Solid Edge part; units mm, degrees
sketch "Sketch1" plane through (0, 0, 0) normal (0, 0, 1) x (1, 0, 0)
  line L0 (0, 0) -> (115, 0)
  line L1 (115, 0) -> (115, 215)
  line L2 (115, 215) -> (0, 215)
  line L3 (0, 215) -> (0, 0)
  dimension "D1" = 115
  dimension "D2" = 0
extrude "Protrusion1" add sketch "Sketch1" along normal blind 30
sketch "Sketch2" plane through (57.5, 107.5, 30) normal (0, 0, 1) x (1, 0, 0)
  circle A0 centre (-20.8, 60.05) radius 30
extrude "ExtrudedCutout_1" cut sketch "Sketch2" against normal blind 2
sketch "Sketch3" plane through (57.5, 107.5, 0) normal (0, 0, -1) x (0, 1, 0)
  circle A0 centre (-75, -25) radius 2
  circle A1 centre (75, -25) radius 2
  circle A2 centre (75, 25) radius 2
  circle A3 centre (-75, 25) radius 2
  dimension "D1" = 75
  dimension "D2" = 75
extrude "ExtrudedCutout_2" cut sketch "Sketch3" against normal blind 3
sketch "Sketch4" plane through (57.5, 107.5, 30) normal (0, 0, 1) x (0, 1, 0)
  line L0 (-107.5, -54.5317) -> (-93.8266, -54.5317)
  line L1 (-93.8266, -54.5317) -> (-93.8266, 35.8867)
  line L2 (-93.8266, 35.8867) -> (-107.5, 35.8867)
  line L3 (-107.5, 35.8867) -> (-107.5, -54.5317)
extrude "ExtrudedCutout_3" cut sketch "Sketch4" against normal blind 11.4081
sketch "Sketch5" plane through (115, 107.5, 15) normal (1, 0, 0) x (0, 1, 0)
  circle A0 centre (-75, -2.5) radius 2
  circle A1 centre (75, -2.5) radius 2
extrude "ExtrudedCutout_4" cut sketch "Sketch5" against normal blind 5
mirror "Mirror1" about plane through (57.5, 0, 0) normal (1, 0, 0) of "ExtrudedCutout_4"
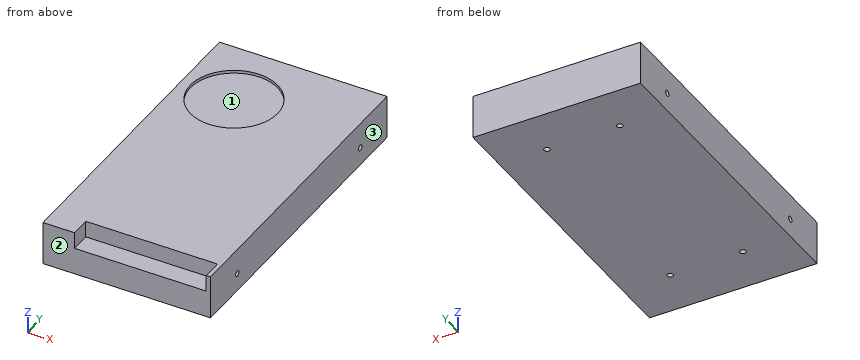
Part model, mm, in its own coordinate system. Face numbers are marked on the shaded views. Round coordinates to 2 decimals unless told otherwise and drop trailing zeros. Write each loop counter-clockwise with the first axis right and the second up, starting at its lowest first coordinate (ties: lowest second). Pieces come first, ordered by that corner, then holes.
Item 1: Cut at A-A, the plane x = 36.7. Give the cut face in (y, z), plus the area to 3 significant figures.
Results:
outline: (0, 0) - (215, 0) - (215, 30) - (197.55, 30) - (197.55, 28) - (137.55, 28) - (137.55, 30) - (13.67, 30) - (13.67, 18.59) - (0, 18.59) - close
area: 6,170 mm2
Item 2: Drop flat-ended pins along their axis: pin 1 Ø1.2 at (y, z) = (31.5, 12.5) entering from +X; pin 2 Ø3 at (x, y) = (32.5, 32.5) entering from -Z; pin 3 Ø11 at (x, y) = (50.5, 4) entering from +Z. Give the stop position or say it passes through.
Results:
pin 1: stops at x = 110
pin 2: stops at z = 3
pin 3: stops at z = 18.59
Item 3: Cut at C-C, the plane x = 76.5. Give the cut face in (y, z), plus the area to 3 significant figures.
Results:
outline: (0, 0) - (215, 0) - (215, 30) - (13.67, 30) - (13.67, 18.59) - (0, 18.59) - close
area: 6,290 mm2
Item 4: Two-plate mould, pull along X, no slides. Class the marked faces 1, 2 and 3: +X half, -X half, draft (parallel to the pull), parting line (faces both ways), or undercut.
Results:
face 1: undercut
face 2: draft
face 3: +X half
Item 5: Cut at B-B, the plane y = 167.55. Give the cut face in (x, z).
Results:
outline: (0, 0) - (115, 0) - (115, 30) - (66.7, 30) - (66.7, 28) - (6.7, 28) - (6.7, 30) - (0, 30) - close
Item 6: Cut at D-D, the plane y = 32.5. Give the cut face in (x, z), plus the area to 3 significant figures.
Results:
outline: (0, 0) - (30.5, 0) - (30.5, 3) - (34.5, 3) - (34.5, 0) - (80.5, 0) - (80.5, 3) - (84.5, 3) - (84.5, 0) - (115, 0) - (115, 10.5) - (110, 10.5) - (110, 14.5) - (115, 14.5) - (115, 30) - (0, 30) - (0, 14.5) - (5, 14.5) - (5, 10.5) - (0, 10.5) - close
area: 3,390 mm2
Item 7: Probe L1, parallel to X at y = 182.5, z = 0.8; L2, parallel to Y at x = 36.7, z = 28.6; L3, parallel to Z at x = 2.7, y = 182.5. List the from-to ranges inside material, lowest first.
Results:
L1: x = 0 to 30.5, 34.5 to 80.5, 84.5 to 115
L2: y = 13.67 to 137.55, 197.55 to 215
L3: z = 0 to 10.5, 14.5 to 30
